Can you work these out from the model? Positions are in its coordinate system, mm. Face numbers are marked on the shaded views. A direction names the side the tool comes from. Give positions to 0.01 mm unless a question says otherwise; leave off trailing zeros. Order: outer loops, then holes, each group sorted by start corner. A loop starts at its lowest first (then second) coordinate and runs counter-clockwise, first axis right, second up. Notation, with made-up numbers: (59.5, -23) - (74.5, -23) arc R15 cw to (74.5, -17) - close; hole circle Ø9 at (22, -16). An arc over 180 degrees is marked (long way). Use one line per item in the form item = value. Start each with the question number.
1) Suppose I cut it at D-D, the plane x = 7. Write out the boundary of the cut face in (y, z), and give its area (3 significant figures).
2) For pin 1 (2 mm diameter, centred on x = 7, z = 39.5, fed in from +Y); pin 2 (4 mm diameter, centred on y = 8.772, z = 41.8, fed in from +X); pin 3 (0.9 mm diameter, centred on x = 1, z = 16.5, fed in from +Y); pin 4 (1.5 mm diameter, centred on y = 8.5, z = 10.5, fed in from -X), each with a flat end and sliding along its axis, tell me the tip position at first contact or that it passes through.
3) Suppose I cut it at C-C, the plane z = 50. Write out the boundary of the cut face in (x, y), and give its area (3 significant figures).
4) We'd pull the mould along Z, two halves only. Please class the marked faces 3, 4, 5 and 6: released by +Z, released by -Z, zero draft, split by the parting line, or undercut.
5) Which directions (+Z, -Z, +X, -X, +Y, -Y) give clear straight access to the entire face, cutting with the end or side of a thin tool? Please do the marked faces 1 and 2.
6) Suppose I cut it at A-A, the plane z = 41.8. Write out the boundary of the cut face in (x, y).
7) Suppose I cut it at B-B, the plane y = 4. Write out the boundary of the cut face in (x, z).
8) Please list where these lines run through material, in increasing order: probe 1 along Y at (x, z) = (12.8, 41.8); probe 2 along X at (y, z) = (9, 52); probe 3 along Y at (x, z) = (9.25, 46.5).
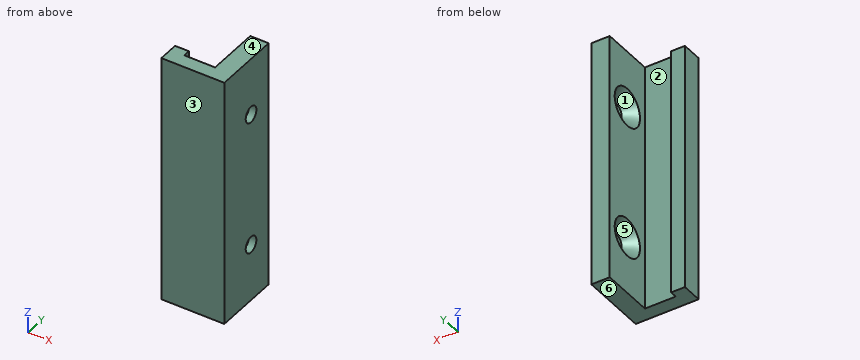
Autodesk Inventor part; units mm, degrees
ref_plane "YZ Plane" through (0, 0, 0) normal (1, 0, 0) x (0, 1, 0)
ref_plane "XZ Plane" through (0, 0, 0) normal (0, 1, 0) x (-1, 0, 0)
ref_plane "XY Plane" through (0, 0, 0) normal (0, 0, 1) x (1, 0, 0)
sketch "Sketch1" plane through (0, 0, 0) normal (0, 0, 1) x (1, 0, 0)
  line L0 (0, 0) -> (0, 4.5)
  line L1 (0, 0) -> (0, 4.5)
  line L2 (0, 4.5) -> (3, 4.5)
  line L3 (0, 4.5) -> (3, 4.5)
  line L4 (3, 4.5) -> (3, 3)
  line L5 (3, 4.5) -> (3, 3)
  line L6 (3, 3) -> (9.7, 3)
  line L7 (3, 3) -> (9.7, 3)
  line L8 (9.7, 3) -> (9.7, 14.544)
  line L9 (9.7, 3) -> (9.7, 14.544)
  line L10 (13.7, 14.544) -> (9.7, 14.544)
  line L11 (9.7, 14.544) -> (13.7, 14.544)
  line L12 (13.7, 14.544) -> (13.7, 0)
  line L13 (13.7, 0) -> (0, 0)
  line L14 (13.7, 0) -> (0, 0)
  point P0 (13.7, 167.0499)
extrude "Extrusion1" add sketch "Sketch1" along normal blind 54.3
sketch "Sketch2" plane through (9.7, 3, 0) normal (-1, 0, 0) x (0, 0, 1)
  circle A0 centre (12.5, 5.772) radius 1.75
  circle A1 centre (41.8, 5.772) radius 1.75
  line L0 (0, 11.544) -> (0, 0)
  line L1 (54.3, 11.544) -> (54.3, 0)
  point P0 (0, -3)
  dimension "d2" = 3.5
  dimension "d3" = 3.5
  dimension "d4" = 12.5
  dimension "d5" = 12.5
extrude "Extrusion2" cut sketch "Sketch2" against normal blind 54.3
chamfer "Chamfer1" distance 2.4 angle 45 2 edges at (9.7, 8.772, 10.75) (9.7, 8.772, 40.05)
equation "\"d5\" = d4"
properties part number "bottomSpacer"
Result sheet:
q1.outline = (0, 0) - (3, 0) - (3, 54.3) - (0, 54.3) - close
q1.area = 163 mm²
q2.pin_1 = 3
q2.pin_2 = 13.7
q2.pin_3 = 4.5
q2.pin_4 = 11.08
q3.outline = (0, 0) - (13.7, 0) - (13.7, 14.54) - (9.7, 14.54) - (9.7, 3) - (3, 3) - (3, 4.5) - (0, 4.5) - close
q3.area = 91.8 mm²
q4.face_3 = zero draft
q4.face_4 = released by +Z
q4.face_5 = undercut
q4.face_6 = released by -Z
q5.face_1 = -X
q5.face_2 = +Z, -Z, +Y
q6.outline = (0, 0) - (13.7, 0) - (13.7, 7.02) - (12.1, 7.02) - (9.7, 4.62) - (9.7, 3) - (3, 3) - (3, 4.5) - (0, 4.5) - close; (9.7, 12.92) - (12.1, 10.52) - (13.7, 10.52) - (13.7, 14.54) - (9.7, 14.54) - close
q7.outline = (0, 0) - (3, 0) - (3, 54.3) - (0, 54.3) - close; (9.7, 0) - (13.7, 0) - (13.7, 54.3) - (9.7, 54.3) - close
q8.probe_1 = 0 to 7.02, 10.52 to 14.54
q8.probe_2 = 9.7 to 13.7
q8.probe_3 = 0 to 3
